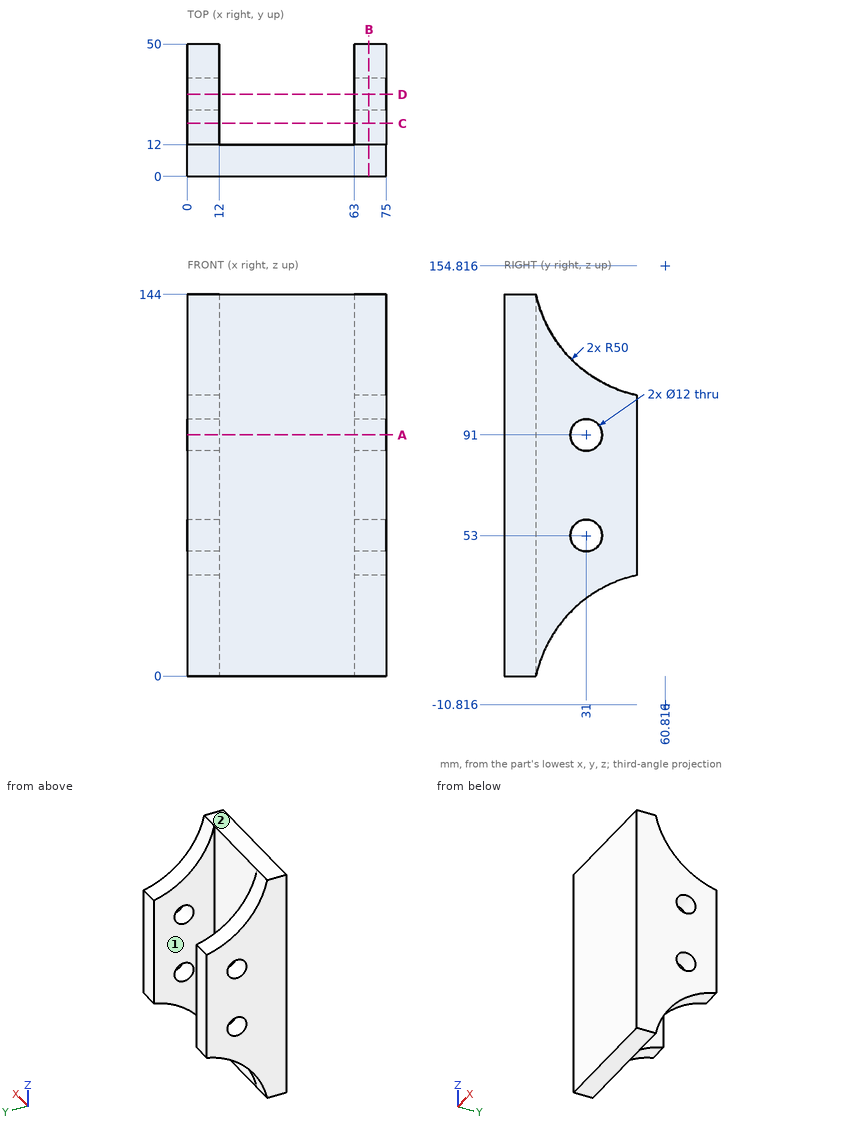
Can you work these out from the drawing? Everything is in mm from the part's minimum corner. A direction names the side the tool comes from. Round coordinates to 2 decimals unless told otherwise and drop trailing zeros. Loops run counter-clockwise (first coordinate to the right, second up) from the corner with the lowest first, then second, coordinate; pieces in that order, holes last. Notation, with made-up numbers: (77.5, 51.25) - (133.5, 51.25) arc R5 cw to (133.5, 55.25) - close; hole circle Ø5 at (67.5, 87). An arc over 180 degrees is marked (long way). Write item = value, one per line. Start each with the question number.
(1) If we section it at D-D (y = 31): Please give me the cut outline in (x, z).
(2) For P1, Ø8, axis at x = 55, z = 101.5, coming from the +Y side; P2, Ø3, axis at x = 10, y = 33, coming from the -Z side, each with a flat end and sliding along its axis, tell me the tip position at first contact or that it passes through.
(3) If I drill on probe 1 along Y at (x, z) = (2.75, 53); probe 2 along X at (y, z) = (47, 73.5); probe 3 along Z at (x, y) = (6, 31), over which ranges is the centre line in solid material (lowest first)? Write a range as [from, to].
(4) If we section it at C-C (y = 20): Please give me the cut outline in (x, z), and give its area (3 significant figures).
(5) If we section it at A-A (z = 91): Please give me the cut outline in (x, y).
(6) If we section it at B-B (x = 68.5): Please give me the cut outline in (y, z).
(7) For the marked faces 1 and 2, which set-ups out of +Z, -Z, +X, -X, +Y, -Y let a thin tool reach every point of the face, with its end or its side?
Ans:
q1.outline = (0, 29.32) - (12, 29.32) - (12, 47) - (0, 47) - close; (0, 59) - (12, 59) - (12, 85) - (0, 85) - close; (0, 97) - (12, 97) - (12, 114.68) - (0, 114.68) - close; (63, 29.32) - (75, 29.32) - (75, 47) - (63, 47) - close; (63, 59) - (75, 59) - (75, 85) - (63, 85) - close; (63, 97) - (75, 97) - (75, 114.68) - (63, 114.68) - close
q2.P1 = 12
q2.P2 = 29.69
q3.probe_1 = [0, 25], [37, 50]
q3.probe_2 = [0, 12], [63, 75]
q3.probe_3 = [29.32, 47], [59, 85], [97, 114.68]
q4.outline = (0, 18.06) - (12, 18.06) - (12, 125.94) - (0, 125.94) - close; (63, 18.06) - (75, 18.06) - (75, 125.94) - (63, 125.94) - close
q4.area = 2,590 mm²
q5.outline = (0, 0) - (75, 0) - (75, 25) - (63, 25) - (63, 12) - (12, 12) - (12, 25) - (0, 25) - close; (0, 37) - (12, 37) - (12, 50) - (0, 50) - close; (63, 37) - (75, 37) - (75, 50) - (63, 50) - close
q6.outline = (0, 0) - (12, 0) arc R50 cw to (50, 38) - (50, 106) arc R50 cw to (12, 144) - (0, 144) - close; hole circle Ø12 at (31, 53); hole circle Ø12 at (31, 91)
q7.face_1 = +Z, -Z, +Y
q7.face_2 = +Z, +X, -X, +Y, -Y
